Autodesk Inventor part; units mm, degrees
ref_plane "YZ Plane" through (0, 0, 0) normal (1, 0, 0) x (0, 1, 0)
ref_plane "XZ Plane" through (0, 0, 0) normal (0, 1, 0) x (-1, 0, 0)
ref_plane "XY Plane" through (0, 0, 0) normal (0, 0, 1) x (1, 0, 0)
sketch "Эскиз1" plane through (0, 0, 0) normal (0, 1, 0) x (-1, 0, 0)
  line L0 (167.5, -227.5) -> (-167.5, -227.5)
  line L1 (-167.5, -227.5) -> (-167.5, 227.5)
  line L2 (-167.5, 227.5) -> (167.5, 227.5)
  line L3 (167.5, 227.5) -> (167.5, -227.5)
  line L4 (167.5, -227.5) -> (-167.5, 227.5) construction
  line L5 (-167.5, -227.5) -> (167.5, 227.5) construction
  point P0 (0, 0)
  dimension "d0" = 335
  dimension "d1" = 455
extrude "Выдавливание1" add sketch "Эскиз1" along normal blind 70
sketch "Эскиз2" plane through (0, 70, 0) normal (0, 1, 0) x (1, 0, 0)
  line L0 (167.5, 227.5) -> (-167.5, 227.5)
  line L1 (-147.5, 227.5) -> (-147.5, -225.4146) construction
  line L2 (-167.5, 227.5) -> (-167.5, -227.5)
  line L3 (-167.5, 207.5) -> (167.5, 207.5)
  line L4 (-167.5, -207.5) -> (167.5, -207.5)
  line L5 (167.5, -227.5) -> (167.5, 227.5)
  line L6 (-167.5, -227.5) -> (167.5, -227.5)
  line L7 (162.5, 227.5) -> (162.5, -227.5)
  line L8 (-147.5, 207.5) -> (-47.5, 207.5)
  line L9 (-47.5, 207.5) -> (-47.5, 107.5)
  line L10 (-47.5, 107.5) -> (-147.5, 107.5)
  line L11 (-147.5, 107.5) -> (-147.5, 207.5)
  line L12 (-42.5, 107.5) -> (-42.5, 207.5)
  line L13 (-42.5, 207.5) -> (57.5, 207.5)
  line L14 (57.5, 207.5) -> (57.5, 107.5)
  line L15 (57.5, 107.5) -> (-42.5, 107.5)
  line L16 (62.5, 107.5) -> (62.5, 207.5)
  line L17 (62.5, 207.5) -> (162.5, 207.5)
  line L18 (162.5, 207.5) -> (162.5, 107.5)
  line L19 (162.5, 107.5) -> (62.5, 107.5)
  line L20 (-147.5, 2.5) -> (-147.5, 102.5)
  line L21 (-147.5, 102.5) -> (-47.5, 102.5)
  line L22 (-47.5, 102.5) -> (-47.5, 2.5)
  line L23 (-47.5, 2.5) -> (-147.5, 2.5)
  line L24 (-42.5, 2.5) -> (-42.5, 102.5)
  line L25 (-42.5, 102.5) -> (57.5, 102.5)
  line L26 (57.5, 102.5) -> (57.5, 2.5)
  line L27 (57.5, 2.5) -> (-42.5, 2.5)
  line L28 (62.5, 2.5) -> (62.5, 102.5)
  line L29 (62.5, 102.5) -> (162.5, 102.5)
  line L30 (162.5, 102.5) -> (162.5, 2.5)
  line L31 (162.5, 2.5) -> (62.5, 2.5)
  line L32 (-147.5, -102.5) -> (-147.5, -2.5)
  line L33 (-147.5, -2.5) -> (-47.5, -2.5)
  line L34 (-47.5, -2.5) -> (-47.5, -102.5)
  line L35 (-47.5, -102.5) -> (-147.5, -102.5)
  line L36 (-42.5, -102.5) -> (-42.5, -2.5)
  line L37 (-42.5, -2.5) -> (57.5, -2.5)
  line L38 (57.5, -2.5) -> (57.5, -102.5)
  line L39 (57.5, -102.5) -> (-42.5, -102.5)
  line L40 (62.5, -102.5) -> (62.5, -2.5)
  line L41 (62.5, -2.5) -> (162.5, -2.5)
  line L42 (162.5, -2.5) -> (162.5, -102.5)
  line L43 (162.5, -102.5) -> (62.5, -102.5)
  line L44 (-147.5, -207.5) -> (-147.5, -107.5)
  line L45 (-147.5, -107.5) -> (-47.5, -107.5)
  line L46 (-47.5, -107.5) -> (-47.5, -207.5)
  line L47 (-47.5, -207.5) -> (-147.5, -207.5)
  line L48 (-42.5, -207.5) -> (-42.5, -107.5)
  line L49 (-42.5, -107.5) -> (57.5, -107.5)
  line L50 (57.5, -107.5) -> (57.5, -207.5)
  line L51 (57.5, -207.5) -> (-42.5, -207.5)
  line L52 (62.5, -207.5) -> (62.5, -107.5)
  line L53 (62.5, -107.5) -> (162.5, -107.5)
  line L54 (162.5, -107.5) -> (162.5, -207.5)
  line L55 (162.5, -207.5) -> (62.5, -207.5)
  point P0 (0, 0)
  point P1 (162.5, -207.5)
  point P2 (162.5, 207.5)
  dimension "d4" = 20
  dimension "d5" = 20
  dimension "d6" = 20
  dimension "d7" = 5
  dimension "d8" = 100
  dimension "d9" = 100
  dimension "d12" = 105
  dimension "d15" = 105
extrude "Выдавливание2" cut sketch "Эскиз2" against normal blind 65 contours L7 L19 L16 L3 | L4 L52 L53 L7 | L3 L9 L10 L11 | L14 L15 L12 L3 | L7 L31 L28 L29 | L44 L45 L46 L4 | L4 L48 L49 L50 | L43 L40 L41 L7 | L20 L21 L22 L23 | L24 L25 L26 L27 | L32 L33 L34 L35 | L36 L37 L38 L39
sketch "Эскиз6" plane through (0, 0, 0) normal (0, -1, 0) x (1, 0, 0)
  line L0 (167.5, -227.5) -> (227.5, -227.5)
  line L1 (227.5, -227.5) -> (227.5, 227.5)
  line L2 (227.5, 227.5) -> (167.5, 227.5)
  line L3 (167.5, 227.5) -> (167.5, -227.5)
  point P0 (0, 0)
  dimension "d29" = 60
extrude "Выдавливание5" add sketch "Эскиз6" against normal blind 70
sketch "Эскиз7" plane through (0, 70, 0) normal (0, 1, 0) x (1, 0, 0)
  line L0 (227.5, 227.5) -> (-167.5, 227.5)
  line L1 (207.5, 227.5) -> (207.5, -226.0922)
  line L2 (227.5, -227.5) -> (227.5, 227.5)
  line L3 (227.5, 207.5) -> (-167.5, 207.5)
  line L4 (207.5, 207.5) -> (167.5, 207.5)
  line L5 (167.5, 207.5) -> (167.5, -207.5)
  line L6 (167.5, -207.5) -> (207.5, -207.5)
  line L7 (207.5, -207.5) -> (207.5, 207.5)
  point P0 (0, 0)
  dimension "d32" = 20
  dimension "d33" = 20
  dimension "d34" = 40
  dimension "d35" = 415
extrude "Выдавливание6" cut sketch "Эскиз7" against normal blind 65 contours L1 L6 L5 L3
ref_plane "РабПлоскость2" through (0, 0, 0) normal (0, -1, 0) x (1, 0, 0)
sketch "Эскиз8" plane through (0, 0, 0) normal (0, -1, 0) x (1, 0, 0)
  point P0 (0, 0)
sketch "Эскиз9" plane through (0, 0, 0) normal (0, -1, 0) x (1, 0, 0)
  line L0 (-167.5, -227.5) -> (-167.5, 227.5)
  line L1 (227.5, -227.5) -> (-167.5, -227.5)
  line L2 (-167.5, 227.5) -> (227.5, 227.5)
  line L3 (227.5, 227.5) -> (227.5, -227.5)
  line L4 (227.5, -227.5) -> (-167.5, -227.5)
  line L5 (-167.5, -227.5) -> (-167.5, 227.5)
  point P0 (0, 0)
sketch "Эскиз10" plane through (0, 0, 0) normal (0, -1, 0) x (1, 0, 0)
  point P0 (0, 0)
sketch "Эскиз11" plane through (0, 0, 0) normal (0, -1, 0) x (1, 0, 0)
  line L0 (-167.5, -227.5) -> (-167.5, 227.5)
  line L1 (227.5, -227.5) -> (-167.5, -227.5)
  line L2 (-167.5, 227.5) -> (227.5, 227.5)
  line L3 (227.5, 227.5) -> (227.5, -227.5)
  line L4 (227.5, -227.5) -> (-167.5, -227.5)
  line L5 (-167.5, -227.5) -> (-167.5, 227.5)
  point P0 (0, 0)
extrude "Выдавливание7" add sketch "Эскиз11" along normal blind 5
sketch "Эскиз12" plane through (0, -5, 0) normal (0, -1, 0) x (1, 0, 0)
  line L0 (-147.5, -229.7416) -> (-147.5, 227.5)
  line L1 (-167.5, 227.5) -> (227.5, 227.5)
  line L2 (-167.5, 227.5) -> (-167.5, -227.5)
  line L3 (-167.5, -207.5) -> (227.5, -207.5)
  line L4 (227.5, 227.5) -> (227.5, -227.5)
  line L5 (-167.5, -227.5) -> (227.5, -227.5)
  line L6 (207.5, 207.5) -> (167.5, 207.5)
  line L7 (-147.5, -207.5) -> (207.5, -207.5)
  line L8 (207.5, -207.5) -> (207.5, 207.5)
  line L9 (207.5, 207.5) -> (-147.5, 207.5)
  line L10 (-147.5, 207.5) -> (-147.5, -207.5)
  point P0 (0, 0)
  dimension "d41" = 20
  dimension "d42" = 20
extrude "Выдавливание8" cut sketch "Эскиз12" against normal blind 5 contours L0 L9 L6 L8 L3
properties part number "ключница"
Can you work these out from the model? Positions are in its coordinate system, mm. Coordinates: 2 decimals unless noted, no trailing zeros. Order: outer loops, then holes, each group sorted by start corner. A loop starts at its lowest first (then second) coordinate and runs counter-clockwise, first axis right, second up. Notation, with made-up numbers: (29, -19.5) -> (86, -19.5) arc R21 cw to (86, -2.5) -> close; hole circle Ø9 at (-34.5, 3.5). An arc over 180 degrees is marked (long way). Use one line per item in the form item = value.
Q1. I need wall thicknesses on L1, parallel to Z at x = 115.5, y = 33; L2, parallel to X at y = 34.5, z = 44; L3, parallel to X at y = 8, z = -1.5. Which ranges of each line are inside material? Lowest first, please.
From the geometry:
L1 = -227.5 to -207.5, -107.5 to -102.5, -2.5 to 2.5, 102.5 to 107.5, 207.5 to 227.5
L2 = -167.5 to -147.5, -47.5 to -42.5, 57.5 to 62.5, 162.5 to 167.5, 207.5 to 227.5
L3 = -167.5 to 167.5, 207.5 to 227.5
Q2. Will these pins go through, and if not, where does the flat tip stop? P1, Ø2, axis at x = 79, z = 26.5, coming from the -Y side; P2, Ø12, axis at x = -30, z = 95.5, coming from the +Y side.
From the geometry:
P1 = 0
P2 = 5
Q3. Imagine slicing it at C-C, the plane y = 59.5. Give the number of separate pieces and of enclosed holes in the cut face, then the cut area to 3 significant figures.
From the geometry:
separate_pieces = 1
enclosed_holes = 13
area = 43,100 mm²
Q4. Imagine slicing it at B-B, the plane z = -191. List the corners of the cut face in (x, y) for me, then the cut area to 3 significant figures.
From the geometry:
outline = (-167.5, -5) -> (-147.5, -5) -> (-147.5, 0) -> (207.5, 0) -> (207.5, -5) -> (227.5, -5) -> (227.5, 70) -> (207.5, 70) -> (207.5, 5) -> (167.5, 5) -> (167.5, 70) -> (162.5, 70) -> (162.5, 5) -> (62.5, 5) -> (62.5, 70) -> (57.5, 70) -> (57.5, 5) -> (-42.5, 5) -> (-42.5, 70) -> (-47.5, 70) -> (-47.5, 5) -> (-147.5, 5) -> (-147.5, 70) -> (-167.5, 70) -> close
area = 5,750 mm²
Q5. Imagine slicing it at D-D, the plane x = 194. List the corners of the cut face in (y, z) for me, then the cut area to 4 significant figures.
From the geometry:
outline = (-5, -227.5) -> (70, -227.5) -> (70, -207.5) -> (5, -207.5) -> (5, 207.5) -> (70, 207.5) -> (70, 227.5) -> (-5, 227.5) -> (-5, 207.5) -> (0, 207.5) -> (0, -207.5) -> (-5, -207.5) -> close
area = 5,075 mm²
Q6. Imagine slicing it at A-A, the plane x = 40.5. List the corners of the cut face in (y, z) for me, then the cut area to 3 significant figures.
From the geometry:
outline = (-5, -227.5) -> (70, -227.5) -> (70, -207.5) -> (5, -207.5) -> (5, -107.5) -> (70, -107.5) -> (70, -102.5) -> (5, -102.5) -> (5, -2.5) -> (70, -2.5) -> (70, 2.5) -> (5, 2.5) -> (5, 102.5) -> (70, 102.5) -> (70, 107.5) -> (5, 107.5) -> (5, 207.5) -> (70, 207.5) -> (70, 227.5) -> (-5, 227.5) -> (-5, 207.5) -> (0, 207.5) -> (0, -207.5) -> (-5, -207.5) -> close
area = 6,050 mm²
Q7. We'd pull the mould along X, two halves only. Please class faces 1 (the face through (-42.5, 38, 53)), 2 (the face through (-161, -5, 1)), 3 (the face through (62.5, 38, 53)): released by +X, released by -X, zero draft, split by the parting line, or undercut.
From the geometry:
face_1 = undercut
face_2 = zero draft
face_3 = undercut
